```python
from build123d import *

# Parameters (mm, degrees)
BOSS_EXTRUDE1_DEPTH = 14


with BuildPart() as part:
    # Sketch1 → Boss-Extrude1 (new body)
    with BuildSketch(Plane.XY):
        with BuildLine():
            Line((-1, 8.440971508), (-1, 11.5))
            Line((-1, 11.5), (1, 11.5))
            Line((1, 11.5), (1, 8.440971508))
            ThreePointArc((1, 8.440971508), (6.01040764, 6.01040764), (8.440971508, 1))
            Line((8.440971508, 1), (11.5, 1))
            Line((11.5, 1), (11.5, -1))
            Line((11.5, -1), (8.440971508, -1))
            ThreePointArc((8.440971508, -1), (6.01040764, -6.01040764), (1, -8.440971508))
            Line((1, -8.440971508), (1, -11.5))
            Line((1, -11.5), (-1, -11.5))
            Line((-1, -11.5), (-1, -8.440971508))
            ThreePointArc((-1, -8.440971508), (-6.01040764, -6.01040764), (-8.440971508, -1))
            Line((-8.440971508, -1), (-11.5, -1))
            Line((-11.5, -1), (-11.5, 1))
            Line((-11.5, 1), (-8.440971508, 1))
            ThreePointArc((-8.440971508, 1), (-6.01040764, 6.01040764), (-1, 8.440971508))
        make_face()
        with BuildLine():
            Line((-1.5, 5.652839314), (-1.5, 7.348469228))
            Line((-1.5, 7.348469228), (1.5, 7.348469228))
            Line((1.5, 7.348469228), (1.5, 5.652839314))
            ThreePointArc((1.5, 5.652839314), (4.135492251, 4.135492251), (5.652839314, 1.5))
            Line((5.652839314, 1.5), (7.348469228, 1.5))
            Line((7.348469228, 1.5), (7.348469228, -1.5))
            Line((7.348469228, -1.5), (5.652839314, -1.5))
            ThreePointArc((5.652839314, -1.5), (4.135492251, -4.135492251), (1.5, -5.652839314))
            Line((1.5, -5.652839314), (1.5, -7.348469228))
            Line((1.5, -7.348469228), (-1.5, -7.348469228))
            Line((-1.5, -7.348469228), (-1.5, -5.652839314))
            ThreePointArc((-1.5, -5.652839314), (-4.135492251, -4.135492251), (-5.652839314, -1.5))
            Line((-5.652839314, -1.5), (-7.348469228, -1.5))
            Line((-7.348469228, -1.5), (-7.348469228, 1.5))
            Line((-7.348469228, 1.5), (-5.652839314, 1.5))
            ThreePointArc((-5.652839314, 1.5), (-4.135492251, 4.135492251), (-1.5, 5.652839314))
        make_face(mode=Mode.SUBTRACT)
    extrude(amount=BOSS_EXTRUDE1_DEPTH)


solid = part.part
```
Model file for the job. Use its own axes, mm. A direction names the side the tool comes from. Coordinates: 2 decimals unless noted, no trailing zeros. Write each loop counter-clockwise with the first axis right and the second up, starting at its lowest first coordinate (ties: lowest second). Pieces come first, ordered by that corner, then holes. Notation, with made-up numbers: (74, 27) - (89, 27) arc R27 cw to (89, 66) - close; hole circle Ø11 at (-16.5, -34.75). An arc over 180 degrees is marked (long way). Use a Markdown table: item, result. Add a question column.
Item 1: Band-saw the part on C-C, the plane y = -2.75. Write the cut outline in (x, z), and give its area (3 significant figures).
Item 2: Drill centre lines: line 1 along X through (y, z) = (0.75, 1.5); line 2 along X through (y, z) = (-7, 3). Where is each one in solid material? Low to high.
Item 3: Band-saw the part on D-D, the plane x = -9.5. Write the cut outline in (y, z).
Item 4: Band-saw the part on A-A, the plane x = 0.5. Write the cut outline in (y, z), and give its area (3 significant figures).
Item 5: Drop flat-ended pins along their axis: pin 1 (0.9 mm diameter, centred on y = -9.5, z = 7, fed in from -X); pin 2 (1.9 mm diameter, centred on y = 6.5, z = 7, fed in from -X); pin 3 (8 mm diameter, centred on x = -4, z = 2, fed in from -Y); pin 4 (1.5 mm diameter, centred on x = 10, z = 4.5, fed in from +Y). Give the stop position or say it passes through.
Item 6: 3-axis set-ups, long thin cutter, end or side, ignore diameter. For faces 1 (the face through (1, 10, 7)), 2 (the face through (-10, -1, 7)), 3 (the face through (1.5, -6, 7)), 4 (the face through (-1, 10, 7)), 5 (the face through (1, -10, 7)): which of +Z, -Z, +X, -X, +Y, -Y reach the whole face in a straight line?
A:
| question | item | result |
|---|---|---|
| 1 | outline | (-8.04, 0) - (-5.16, 0) - (-5.16, 14) - (-8.04, 14) - close; (5.16, 0) - (8.04, 0) - (8.04, 14) - (5.16, 14) - close |
| 1 | area | 80.7 mm² |
| 2 | line 1 | x = -11.5 to -7.35, 7.35 to 11.5 |
| 2 | line 2 | x = -4.82 to -1.5, 1.5 to 4.82 |
| 3 | outline | (-1, 0) - (1, 0) - (1, 14) - (-1, 14) - close |
| 4 | outline | (-11.5, 0) - (-7.35, 0) - (-7.35, 14) - (-11.5, 14) - close; (7.35, 0) - (11.5, 0) - (11.5, 14) - (7.35, 14) - close |
| 4 | area | 116 mm² |
| 5 | pin 1 | stops at x = -1 |
| 5 | pin 2 | stops at x = -6.44 |
| 5 | pin 3 | stops at y = -11.5 |
| 5 | pin 4 | stops at y = 1 |
| 6 | face 1 | +Z, -Z, +X, +Y |
| 6 | face 2 | +Z, -Z, -X, -Y |
| 6 | face 3 | +Z, -Z |
| 6 | face 4 | +Z, -Z, -X, +Y |
| 6 | face 5 | +Z, -Z, +X, -Y |
